Could you check a few things on this model? Use its own coordinates, in mm. Round coordinates to 2 decimals unless told otherwise and drop trailing zeros. Order: outer loops, then holes, each group sorted by start corner. A loop starts at its lowest first (then second) coordinate and runs counter-clockwise, first axis right, second up. Notation, with made-up numbers: M -25,61.5 L 12,61.5 A33 ccw 12,96.5 Z; hole C 48,31.25 d7. An arc over 180 degrees is marked long. Write each question's results on one line, items separated by ' | '. Start each with the question number.
1. Please list where these lines run through material, in increasing order: L1, parallel to X at y = -24.5, z = -1; L2, parallel to Y at x = 23.5, z = 12; L3, parallel to X at y = -24, z = -21.
2. I'm going to push flat-ended pins straight in: pin 1 (3 mm diameter, centred on x = 22.5, z = 11.5, fed in from -Y); pin 2 (1 mm diameter, centred on x = 20.5, z = 4, fed in from +Y). Where does each tip first touch, or does it pass through?
3. Suppose I cut it at A-A on z = 9. Write out the boundary of the cut face in (x, y), and give its area (3 significant figures).
from build123d import *

# Parameters (mm, degrees)
F0_W     = 58.7931647897
F0_H     = 58.7931647897
F1_DEPTH = 12.7
F2_W     = 58.7931647897
F2_H     = 16.6965823948
F2_H_2   = 25.4
F3_DEPTH = 58.7931647897
F4_SIZE  = 12.7


with BuildPart() as f1:
    # F0 (on Top) → F1 (new body, symmetric)
    with BuildSketch(Plane.XY):
        Rectangle(F0_W, F0_H)
    extrude(amount=F1_DEPTH, both=True)

    # F2 (on face) → F3 (join, through all)
    with BuildSketch(Plane.XZ.offset(29.3965823948)):
        with Locations((0, 21.0482911974)):
            Rectangle(F2_W, F2_H)
        with Locations((0, -21.0482911974)):
            Rectangle(F2_W, F2_H)
        Rectangle(F2_W, F2_H_2)
    extrude(amount=-F3_DEPTH)

    # F4
    f4_edges = [f1.edges().sort_by_distance(p)[0] for p in [
        (0, 29.396582, 29.396582),
        (-29.396582, 0, 29.396582),
        (-29.396582, 29.396582, 0),
        (29.396582, 0, 29.396582),
        (0, -29.396582, 29.396582),
        (0, 29.396582, -29.396582),
        (29.396582, 29.396582, 0),
        (-29.396582, -29.396582, 0),
        (-29.396582, 0, -29.396582),
        (0, -29.396582, -29.396582),
        (29.396582, -29.396582, 0),
        (29.396582, 0, -29.396582),
    ]]
    chamfer(f4_edges, length=F4_SIZE)


solid = f1.part
Filled sheet:
1) L1: x = -21.59 to 21.59 | L2: y = -22.59 to 22.59 | L3: x = -17.79 to 17.79
2) pin 1: stops at y = -25.09 | pin 2: stops at y = 26.09
3) outline: M -29.4,-16.7 L -16.7,-29.4 L 16.7,-29.4 L 29.4,-16.7 L 29.4,16.7 L 16.7,29.4 L -16.7,29.4 L -29.4,16.7 Z | area: 3,130 mm^2
